The figure shows three views and two pictorial views of one solid part (mm, origin at its lowest corner). Answer the questions. A direction names the side the tool comes from. Round coordinates to 2 decimals unless told otherwise and drop trailing zeros. Order: outer loops, then holes, each group sorted by start corner. A loop starts at its lowest first (then second) coordinate and runs counter-clockwise, first axis right, second up. Notation, with made-up numbers: (35.5, 50.5) - (39.5, 50.5) arc R12 cw to (39.5, 54.5) - close; hole circle Ø3 at (31.25, 51.25). An arc over 180 degrees is marked (long way). Answer as a JSON object with one key per item and string values. Group by question number.
Q1. A cutting plane is placed at D-D on x = 17.5. Determine the outline of the cut face in (y, z), and give its area (3 significant figures).
Q2. A cutting plane is placed at B-B on x = 11. Determine the outline of the cut face in (y, z), and give its area (3 significant figures).
Q3. The mould has two halves that part along X. Classify the marked faces 3, 4 and 5: pulls with the +X half, pulls with the -X half, needs draft (parallel to the pull), parting line crosses it, or undercut.
Q4. Consider line 1 (Z direction, x = 4.5, y = 12.5); line 2 (Z direction, x = 9.25, y = 11.5) (1 decimal); line 3 (X direction, y = 9, z = 8.75) (1 decimal). Determine where each line is inside the solid, lowest interval first.
Q5. A cutting plane is placed at C-C on y = 15. Determine the outline of the cut face in (x, z), and give its area (3 significant figures).
Q6. Given pin 1 Ø1.5 at (y, z) = (13, 2.5) entering from +X; pin 2 Ø8 at (x, y) = (17.5, 13) entering from +Z; pin 3 Ø2 at (x, y) = (15.5, 10.5) entering from +Z; pin 4 Ø8 at (x, z) = (11, 11) entering from +Y, each flat-ended and moving along its own axis, determine where each tip first touches the part or whether it passes through.
Q7. A tool of negligible diameter and unlimited length cuts with its end or side. For the marked faces 1 and 2, from which of +Z, -Z, +X, -X, +Y, -Y can it reach the whole face along a straight path? Write none if from no direction.
Q8. A cutting plane is placed at A-A on z = 11. Determine the outline of the cut face in (x, y).
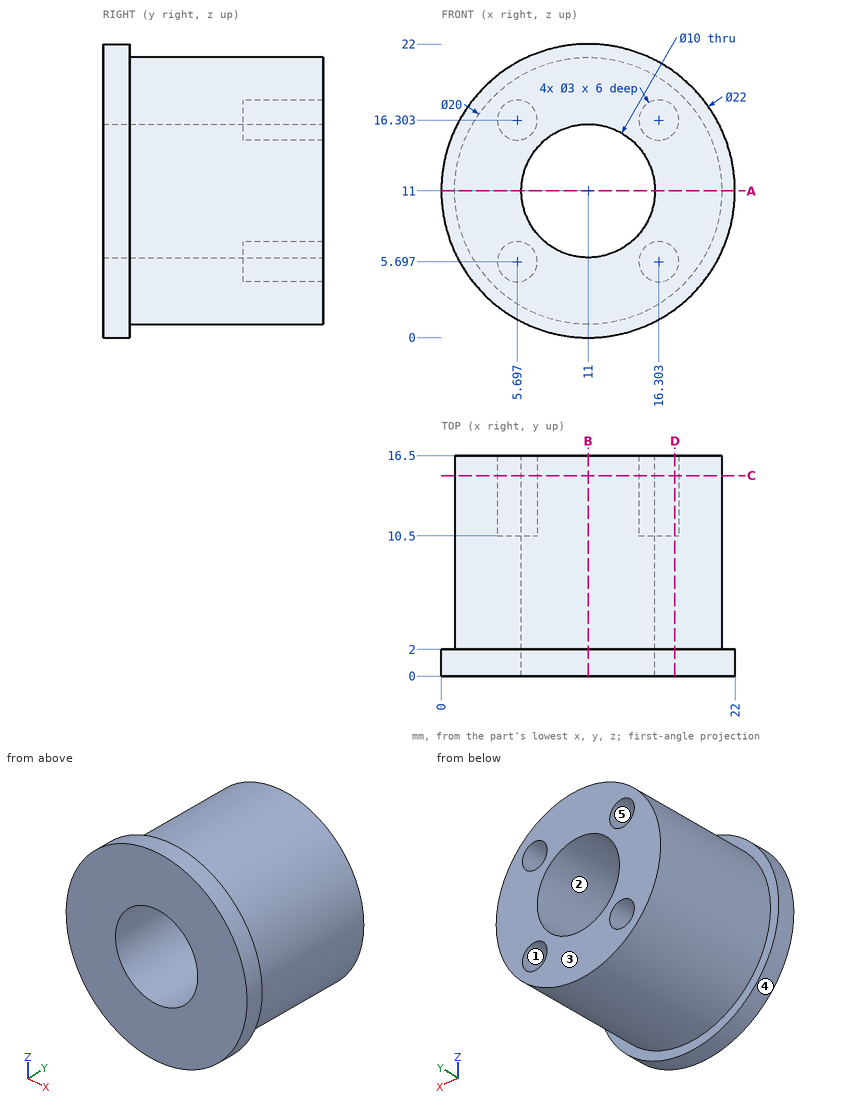
Result set:
{
 "1": {"outline": "(0, 2.13) - (2, 2.13) - (2, 3.4) - (16.5, 3.4) - (16.5, 4.79) - (10.5, 4.79) - (10.5, 6.6) - (16.5, 6.6) - (16.5, 15.4) - (10.5, 15.4) - (10.5, 17.21) - (16.5, 17.21) - (16.5, 18.6) - (2, 18.6) - (2, 19.87) - (0, 19.87) - close", "area": "234 mm²"},
 "2": {"outline": "(0, 0) - (2, 0) - (2, 1) - (16.5, 1) - (16.5, 6) - (0, 6) - close; (0, 16) - (16.5, 16) - (16.5, 21) - (2, 21) - (2, 22) - (0, 22) - close", "area": "169 mm²"},
 "3": {"face 3": "needs draft", "face 4": "parting line crosses it", "face 5": "undercut"},
 "4": {"line 1": "z = 3.4 to 4.79, 6.6 to 15.4, 17.21 to 18.6", "line 2": "z = 1.2 to 6.3, 15.7 to 20.8", "line 3": "x = 1.3 to 6.5, 15.5 to 20.7"},
 "5": {"outline": "circle Ø20 at (11, 11); hole circle Ø3 at (5.7, 5.7); hole circle Ø3 at (5.7, 16.3); hole circle Ø10 at (11, 11); hole circle Ø3 at (16.3, 5.7); hole circle Ø3 at (16.3, 16.3)", "area": "207 mm²"},
 "6": {"pin 1": "stops at x = 17.32", "pin 2": "stops at z = 20.68", "pin 3": "stops at z = 20.37", "pin 4": "passes through"},
 "7": {"face 1": "+Y", "face 2": "+Y, -Y"},
 "8": {"outline": "(0, 0) - (6, 0) - (6, 16.5) - (1, 16.5) - (1, 2) - (0, 2) - close; (16, 0) - (22, 0) - (22, 2) - (21, 2) - (21, 16.5) - (16, 16.5) - close"}
}
